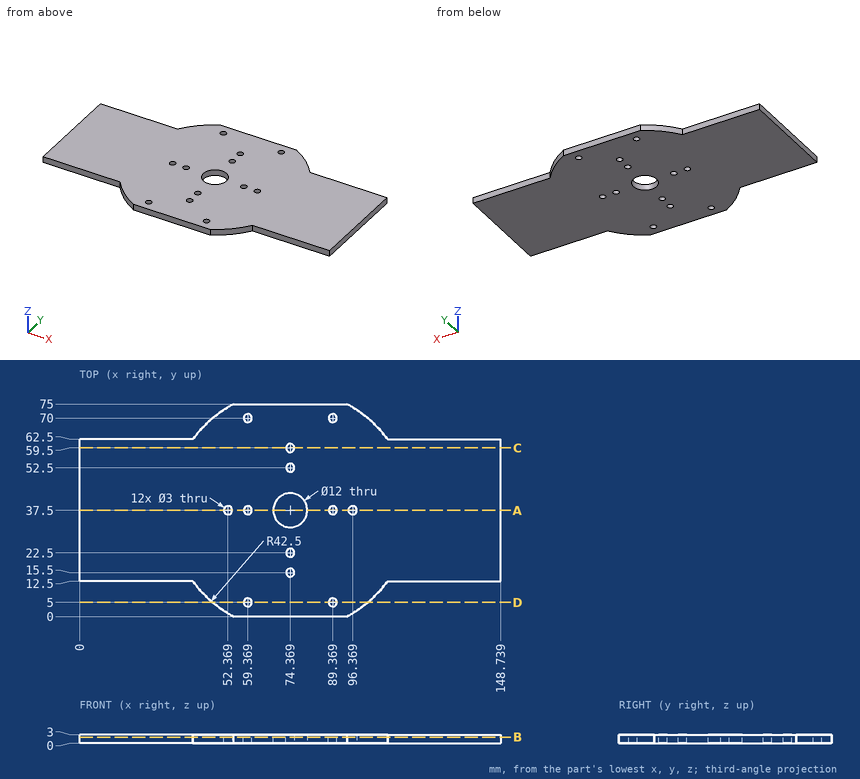
The figure shows three views and two pictorial views of one solid part (mm, origin at its lowest corner). Answer the questions. Give positions to 0.01 mm unless a question says otherwise; leave off trailing zeros. Order: outer loops, then holes, each group sorted by start corner. A loop starts at its lowest first (then second) coordinate and runs counter-clockwise, first axis right, second up. Notation, with made-up numbers: (17, 2) -> (68, 2) arc R24 cw to (68, 31) -> close; hole circle Ø7 at (7.25, 45.5). An arc over 180 degrees is marked (long way). One line per item, written item: value.
1) Flat-ended cylindrical pins translate along their axes: P1, Ø1.5, axis at x = 14.5, z = 2, coming from the +Y side; P2, Ø2.5, axis at x = 59.37, y = 70, coming from the -Z side; P3, Ø1.5, axis at x = 124, z = 1, coming from the -Y side. Find the tip coordinate at first contact, or state that the pin passes through.
Reported:
P1: stops at y = 62.5
P2: passes through
P3: stops at y = 12.5
2) Find the intervals of material crossed by line 1 (X direction, y = 15.5, z = 1.65); line 2 (Y direction, x = 138.5, z = 0.5); line 3 (Y direction, x = 103.5, z = 0.4) (1 decimal), in increasing order.
Reported:
line 1: x = 0 to 72.87, 75.87 to 148.74
line 2: y = 12.5 to 62.5
line 3: y = 6.6 to 68.4
3) Find section D-D, the plane y = 5. Determine the outline of the cut face in (x, z) (1 decimal).
Reported:
outline: (47, 0) -> (57.9, 0) -> (57.9, 3) -> (47, 3) -> close; (60.9, 0) -> (87.9, 0) -> (87.9, 3) -> (60.9, 3) -> close; (90.9, 0) -> (101.8, 0) -> (101.8, 3) -> (90.9, 3) -> close
4) Find section C-C, the plane y = 59.5. Determine the outline of the cut face in (x, z), plus the area to 3 significant figures.
Reported:
outline: (0, 0) -> (72.87, 0) -> (72.87, 3) -> (0, 3) -> close; (75.87, 0) -> (148.74, 0) -> (148.74, 3) -> (75.87, 3) -> close
area: 437 mm^2
5) Find section B-B, the plane z = 2.05. Count the separate pieces of the cut face and the enclosed holes in it, plus the area to 3 significant figures.
Reported:
separate pieces: 1
enclosed holes: 13
area: 8,650 mm^2
6) Find section A-A, the plane y = 37.5. Determine the outline of the cut face in (x, z), plus the area to 3 significant figures.
Reported:
outline: (0, 0) -> (50.87, 0) -> (50.87, 3) -> (0, 3) -> close; (53.87, 0) -> (57.87, 0) -> (57.87, 3) -> (53.87, 3) -> close; (60.87, 0) -> (68.37, 0) -> (68.37, 3) -> (60.87, 3) -> close; (80.37, 0) -> (87.87, 0) -> (87.87, 3) -> (80.37, 3) -> close; (90.87, 0) -> (94.87, 0) -> (94.87, 3) -> (90.87, 3) -> close; (97.87, 0) -> (148.74, 0) -> (148.74, 3) -> (97.87, 3) -> close
area: 374 mm^2
